Could you check a few things on this model? Use its own coordinates, in mm. Face numbers are marked on the shaded views. A direction names the side the tool comes from. Give positions to 0.01 mm unless a question says otherwise; leave off trailing zeros. Loops run counter-clockwise (first coordinate to the right, second up) from the corner with the lowest first, then second, coordinate; pieces in that order, holes last. Notation, with made-up numbers: M -27,26.5 L -12,26.5 A32 ccw -12,58.5 Z; hole C 80.25,9.5 d2. An arc over 180 degrees is marked long. Use a Markdown table: item, result. Add a question column.
1) Suppose I cut it at A-A on x = 5.25. List the corners of the cut face in (y, z) for me, and give its area (3 significant figures).
2) We'd pull the mould along X, two halves only. Please class the marked faces 6, 7 and 8: +X half, -X half, draft (parallel to the pull), parting line (faces both ways), or undercut.
3) Will these pins go through, and if not, where does the flat tip stop? pin 1 Ø3 at (x, z) = (0.63, -3.28) entering from -Y; pin 2 Ø2 at (x, y) = (6, 6) entering from -Z; pin 3 Ø1.5 at (x, y) = (-5.5, 3) entering from +Z.
4) Which directions (+Z, -Z, +X, -X, +Y, -Y) give clear straight access to the entire face, cutting with the end or side of a thin tool? Please do the marked faces 1, 2, 3, 4 and 5.
5) If I drill on line 1 along Z through (x, y) = (12, 1.5); line 2 along Z through (x, y) = (10.5, 1.25); line 3 along X through (y, z) = (4.5, -3.5), over which ranges is the centre line in solid material (lowest first)? Write a range as [from, to].
6) Suppose I cut it at B-B on y = 6.5. List the corners of the cut face in (x, z) for me.
```python
from build123d import *

# Parameters (mm, degrees)
BOSS_EXTRUDE1_DEPTH = 4
SKETCH2_R           = 5
BOSS_EXTRUDE2_DEPTH = 3.5
SKETCH3_R           = 2.7
CUT_EXTRUDE1_DEPTH  = 3.4
SKETCH4_R           = 2.35
CUT_EXTRUDE2_DEPTH  = 1.5


with BuildPart() as part:
    # Sketch1 → Boss-Extrude1 (new body)
    with BuildSketch(Plane(origin=(0, 0, 0), x_dir=(1, 0, 0), z_dir=(0, 1, 0))):
        with BuildLine():
            ThreePointArc((3.901208796, 14.038686533), (3.966253303, 15.234612101), (3.74502345, 16.41169583))
            ThreePointArc((3.74502345, 16.41169583), (3.4723799, 16.473432267), (3.198516489, 16.529510113))
            ThreePointArc((3.198516489, 16.529510113), (2.511969944, 15.548122017), (2.078508173, 14.431618705))
            ThreePointArc((2.078508173, 14.431618705), (1.601109064, 14.483383768), (1.121935684, 14.514727092))
            ThreePointArc((1.121935684, 14.514727092), (0.887522104, 15.689256371), (0.380513774, 16.774342223))
            ThreePointArc((0.380513774, 16.774342223), (0.101082595, 16.766335403), (-0.178122887, 16.752544399))
            ThreePointArc((-0.178122887, 16.752544399), (-0.599039015, 15.631251232), (-0.741219705, 14.442027366))
            ThreePointArc((-0.741219705, 14.442027366), (-1.216493891, 14.373441804), (-1.688407925, 14.284634846))
            ThreePointArc((-1.688407925, 14.284634846), (-2.207550525, 15.363967841), (-2.968480134, 16.288875881))
            ThreePointArc((-2.968480134, 16.288875881), (-3.237141254, 16.211628901), (-3.504145299, 16.128835588))
            ThreePointArc((-3.504145299, 16.128835588), (-3.632983302, 14.938092323), (-3.474949175, 13.750871212))
            ThreePointArc((-3.474949175, 13.750871212), (-3.918235212, 13.566244507), (-4.353237807, 13.362867335))
            ThreePointArc((-4.353237807, 13.362867335), (-5.124489789, 14.279185585), (-6.091528671, 14.985800439))
            ThreePointArc((-6.091528671, 14.985800439), (-6.332538765, 14.844167012), (-6.570564527, 14.697573597))
            ThreePointArc((-6.570564527, 14.697573597), (-6.399229039, 13.512199013), (-5.95090996, 12.401578126))
            ThreePointArc((-5.95090996, 12.401578126), (-6.334354558, 12.112511054), (-6.7051129, 11.807342604))
            ThreePointArc((-6.7051129, 11.807342604), (-7.680013665, 12.503070462), (-8.792399211, 12.946992921))
            ThreePointArc((-8.792399211, 12.946992921), (-8.990614728, 12.749872395), (-9.184706174, 12.548689882))
            ThreePointArc((-9.184706174, 12.548689882), (-8.723962833, 11.443165424), (-8.013528339, 10.478929154))
            ThreePointArc((-8.013528339, 10.478929154), (-8.313038262, 10.103584863), (-8.596256242, 9.71579999))
            ThreePointArc((-8.596256242, 9.71579999), (-9.713549189, 10.147222317), (-10.901386124, 10.3005591))
            ThreePointArc((-10.901386124, 10.3005591), (-11.044352455, 10.060337283), (-11.182314104, 9.817206709))
            ThreePointArc((-11.182314104, 9.817206709), (-10.46111311, 8.860996544), (-9.533202414, 8.103731404))
            ThreePointArc((-9.533202414, 8.103731404), (-9.729958352, 7.665694155), (-9.907840342, 7.21965881))
            ThreePointArc((-9.907840342, 7.21965881), (-11.097321846, 7.359667754), (-12.285974007, 7.212784147))
            ThreePointArc((-12.285974007, 7.212784147), (-12.364708051, 6.944555059), (-12.437871267, 6.674753212))
            ThreePointArc((-12.437871267, 6.674753212), (-11.50152833, 5.927939542), (-10.414445472, 5.425227285))
            ThreePointArc((-10.414445472, 5.425227285), (-10.496084526, 4.952020569), (-10.557453547, 4.475760793))
            ThreePointArc((-10.557453547, 4.475760793), (-11.744384111, 4.315559077), (-12.85916411, 3.877684317))
            ThreePointArc((-12.85916411, 3.877684317), (-12.868718719, 3.598301779), (-12.872486386, 3.318781301))
            ThreePointArc((-12.872486386, 3.318781301), (-11.779835377, 2.828289175), (-10.601885772, 2.611717061))
            ThreePointArc((-10.601885772, 2.611717061), (-10.563278261, 2.133074197), (-10.504278271, 1.656515143))
            ThreePointArc((-10.504278271, 1.656515143), (-11.614078682, 1.206168831), (-12.584940793, 0.504816199))
            ThreePointArc((-12.584940793, 0.504816199), (-12.524715614, 0.231834843), (-12.458850997, -0.039840966))
            ThreePointArc((-12.458850997, -0.039840966), (-11.278547197, -0.243192124), (-10.08374575, -0.160016072))
            ThreePointArc((-10.08374575, -0.160016072), (-9.927317525, -0.614020193), (-9.751655711, -1.060934567))
            ThreePointArc((-9.751655711, -1.060934567), (-10.714593128, -1.773128561), (-11.480534513, -2.693890499))
            ThreePointArc((-11.480534513, -2.693890499), (-11.354313716, -2.943318251), (-11.222955331, -3.190079))
            ThreePointArc((-11.222955331, -3.190079), (-10.029161569, -3.093511889), (-8.89258205, -2.715813928))
            ThreePointArc((-8.89258205, -2.715813928), (-8.628162071, -3.116652557), (-8.34687591, -3.505840978))
            ThreePointArc((-8.34687591, -3.505840978), (-9.102445434, -4.435132885), (-9.61533918, -5.517449271))
            ThreePointArc((-9.61533918, -5.517449271), (-9.431053682, -5.727650955), (-9.242455259, -5.93399176))
            ThreePointArc((-9.242455259, -5.93399176), (-8.110181987, -5.543574046), (-7.103239867, -4.895086329))
            ThreePointArc((-7.103239867, -4.895086329), (-6.747442615, -5.217573301), (-6.378206351, -5.524581628))
            ThreePointArc((-6.378206351, -5.524581628), (-6.87893277, -6.61258062), (-7.106551876, -7.788445534))
            ThreePointArc((-7.106551876, -7.788445534), (-6.875781012, -7.946213407), (-6.641792884, -8.099169115))
            ThreePointArc((-6.641792884, -8.099169115), (-5.642184996, -7.43943218), (-4.828150152, -6.560901574))
            ThreePointArc((-4.828150152, -6.560901574), (-4.403331676, -6.784773846), (-3.969345782, -6.990311618))
            ThreePointArc((-3.969345782, -6.990311618), (-4.183766613, -8.168654718), (-4.111808933, -9.364184243))
            ThreePointArc((-4.111808933, -9.364184243), (-3.849052886, -9.459605167), (-3.584377387, -9.54956501))
            ThreePointArc((-3.584377387, -9.54956501), (-2.780243924, -8.661962551), (-2.210265158, -7.608590366))
            ThreePointArc((-2.210265158, -7.608590366), (-1.743118366, -7.71978122), (-1.271651772, -7.810933742))
            ThreePointArc((-1.271651772, -7.810933742), (-1.186294165, -9.005581318), (-0.819281066, -10.145655938))
            ThreePointArc((-0.819281066, -10.145655938), (-0.541049764, -10.172734267), (-0.26231743, -10.194045736))
            ThreePointArc((-0.26231743, -10.194045736), (0.295814947, -9.134349079), (0.585923772, -7.972322564))
            ThreePointArc((0.585923772, -7.972322564), (1.06604633, -7.96384547), (1.545369644, -7.934885294))
            ThreePointArc((1.545369644, -7.934885294), (1.925142356, -9.070773246), (2.564150092, -10.083757879))
            ThreePointArc((2.564150092, -10.083757879), (2.840374352, -10.040792181), (3.115649745, -9.992116198))
            ThreePointArc((3.115649745, -9.992116198), (3.392711524, -8.826909983), (3.384721804, -7.629243537))
            ThreePointArc((3.384721804, -7.629243537), (3.847652261, -7.501631141), (4.304714649, -7.354377941))
            ThreePointArc((4.304714649, -7.354377941), (4.95503995, -8.360134252), (5.825891117, -9.182379348))
            ThreePointArc((5.825891117, -9.182379348), (6.082752149, -9.072069317), (6.337274035, -8.956464373))
            ThreePointArc((6.337274035, -8.956464373), (6.315856407, -7.758962791), (6.010270165, -6.600910201))
            ThreePointArc((6.010270165, -6.600910201), (6.426920898, -6.362180861), (6.833003449, -6.105887097))
            ThreePointArc((6.833003449, -6.105887097), (7.713019008, -6.918316398), (8.760994824, -7.498157274))
            ThreePointArc((8.760994824, -7.498157274), (8.982353106, -7.327434094), (9.200128938, -7.152164073))
            ThreePointArc((9.200128938, -7.152164073), (8.881577651, -5.997610553), (8.297595995, -4.951936522))
            ThreePointArc((8.297595995, -4.951936522), (8.641787307, -4.617090479), (8.97137436, -4.267860032))
            ThreePointArc((8.97137436, -4.267860032), (10.025785563, -4.835914403), (11.185037854, -5.136917523))
            ThreePointArc((11.185037854, -5.136917523), (11.35698463, -4.91650836), (11.524330752, -4.692586122))
            ThreePointArc((11.524330752, -4.692586122), (10.928661555, -3.653525508), (10.1029782, -2.785933582))
            ThreePointArc((10.1029782, -2.785933582), (10.353083284, -2.376010444), (10.585465673, -1.955786746))
            ThreePointArc((10.585465673, -1.955786746), (11.748019987, -2.243773242), (12.945708667, -2.247025474))
            ThreePointArc((12.945708667, -2.247025474), (13.057439889, -1.990779446), (13.163841329, -1.732274849))
            ThreePointArc((13.163841329, -1.732274849), (12.328482308, -0.873995139), (11.312977976, -0.238999309))
            ThreePointArc((11.312977976, -0.238999309), (11.45328181, 0.220243944), (11.573858095, 0.685056692))
            ThreePointArc((11.573858095, 0.685056692), (12.771507956, 0.695233323), (13.932377842, 0.989936328))
            ThreePointArc((13.932377842, 0.989936328), (13.976873026, 1.265918341), (14.01564419, 1.542762503))
            ThreePointArc((14.01564419, 1.542762503), (12.993084025, 2.166332436), (11.851566587, 2.528833047))
            ThreePointArc((11.851566587, 2.528833047), (11.873253365, 3.008540473), (11.874447295, 3.488736377))
            ThreePointArc((11.874447295, 3.488736377), (13.031939958, 3.796436699), (14.083049324, 4.370577669))
            ThreePointArc((14.083049324, 4.370577669), (14.057512675, 4.648954702), (14.026217428, 4.926743291))
            ThreePointArc((14.026217428, 4.926743291), (12.880707334, 5.276422256), (11.68490253, 5.343650401))
            ThreePointArc((11.68490253, 5.343650401), (11.586609593, 5.813680219), (11.468346148, 6.279086803))
            ThreePointArc((11.468346148, 6.279086803), (12.512952092, 6.864976874), (13.388255872, 7.682480419))
            ThreePointArc((13.388255872, 7.682480419), (13.29429195, 7.945761019), (13.194896688, 8.207039558))
            ThreePointArc((13.194896688, 8.207039558), (11.998413278, 8.260855939), (10.823457921, 8.028587426))
            ThreePointArc((10.823457921, 8.028587426), (10.611361374, 8.459405933), (10.381071482, 8.880779992))
            ThreePointArc((10.381071482, 8.880779992), (11.247154274, 9.708046183), (11.891653912, 10.717545549))
            ThreePointArc((11.891653912, 10.717545549), (11.735166817, 10.949186827), (11.573916909, 11.177538224))
            ThreePointArc((11.573916909, 11.177538224), (10.401639636, 10.932110541), (9.321360492, 10.414939655))
            ThreePointArc((9.321360492, 10.414939655), (9.008787143, 10.77947694), (8.680940764, 11.13034199))
            ThreePointArc((8.680940764, 11.13034199), (9.314081237, 12.147004125), (9.68728045, 13.285068754))
            ThreePointArc((9.68728045, 13.285068754), (9.478102841, 13.470515838), (9.265130213, 13.651591934))
            ThreePointArc((9.265130213, 13.651591934), (8.190717569, 13.12234131), (7.27299255, 12.3527638))
            ThreePointArc((7.27299255, 12.3527638), (6.879582531, 12.628114645), (6.474779459, 12.886424546))
            ThreePointArc((6.474779459, 12.886424546), (6.835195068, 14.028602002), (6.913644378, 15.223723109))
            ThreePointArc((6.913644378, 15.223723109), (6.664919654, 15.351323676), (6.413606158, 15.473746794))
            ThreePointArc((6.413606158, 15.473746794), (5.504567441, 14.693927992), (4.807060586, 13.720299244))
            ThreePointArc((4.807060586, 13.720299244), (4.357533295, 13.889162343), (3.901208796, 14.038686533))
        make_face()
    extrude(amount=BOSS_EXTRUDE1_DEPTH)

    # Sketch2 → Boss-Extrude2 (add)
    with BuildSketch(Plane(origin=(0, 4, 0), x_dir=(1, 0, 0), z_dir=(0, 1, 0))):
        with Locations((0.627447718, 3.276600796)):
            Circle(SKETCH2_R)
    extrude(amount=BOSS_EXTRUDE2_DEPTH)

    # Sketch3 → Cut-Extrude1 (cut)
    with BuildSketch(Plane(origin=(0, 7.5, 0), x_dir=(1, 0, 0), z_dir=(0, 1, 0))):
        with Locations((0.627447718, 3.276600796)):
            Circle(SKETCH3_R)
    extrude(amount=-CUT_EXTRUDE1_DEPTH, mode=Mode.SUBTRACT)

    # Sketch4 → Cut-Extrude2 (cut)
    with BuildSketch(Plane.XZ):
        with Locations((0.627447718, -3.276600796)):
            Circle(SKETCH4_R)
    extrude(amount=-CUT_EXTRUDE2_DEPTH, mode=Mode.SUBTRACT)


solid = part.part
```
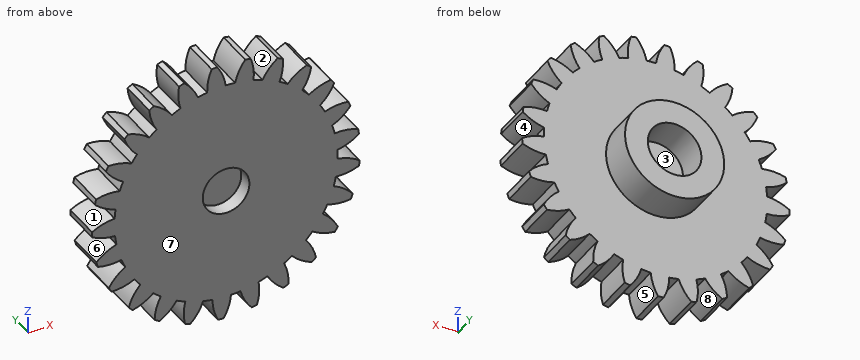
Answer block:
| question | item | result |
|---|---|---|
| 1 | outline | M 0,-14.39 L 4,-14.39 L 4,-5.18 L 7.5,-5.18 L 7.5,-1.37 L 4,-1.37 L 4,8.68 L 0,8.68 Z |
| 1 | area | 106 mm^2 |
| 2 | face 6 | -X half |
| 2 | face 7 | draft |
| 2 | face 8 | undercut |
| 3 | pin 1 | stops at y = 1.5 |
| 3 | pin 2 | stops at z = -5.7 |
| 3 | pin 3 | stops at z = 7.88 |
| 4 | face 1 | -X, +Y, -Y |
| 4 | face 2 | +Z, +Y, -Y |
| 4 | face 3 | +Y |
| 4 | face 4 | +X, +Y, -Y |
| 4 | face 5 | -Z, +Y, -Y |
| 5 | line 1 | z = [-8.26, -6.54], [-5.35, -3.51], [-2.5, -0.66], [0.63, 2.27] |
| 5 | line 2 | z = [-10.96, -8.97], [-8.67, 2.12], [3.15, 5] |
| 5 | line 3 | x = [-4.37, -2.06], [3.32, 5.62] |
| 6 | outline | C 0.63,-3.28 d10; hole C 0.63,-3.28 d5.4 |
